Work out the finished part from the listing and answer in its coordinate system (mm). A direction names the side the tool comes from. Round coordinates to 2 decimals unless told otherwise and drop trailing zeros. Loops run counter-clockwise (first coordinate to the right, second up) from the corner with the lowest first, then second, coordinate; pieces in that order, holes last.
from build123d import *

# Parameters (mm, degrees)
F3_D = 6.3
F5_D = 6.3


with BuildPart() as f1:
    # F0 (on Front) → F1 (revolve)
    with BuildSketch(Plane.XZ):
        Polygon((-47.65, 6.3), (-47.65, 0), (-3.15, 0), (-3.15, 12.6), (-49.55, 12.6), (-49.55, 6.3), align=None)
    revolve(axis=Axis((0, 0, -5.1516543608), (0, 0, -1)))

    # F3 (through all)
    with Locations(Plane(origin=(0, 0, 0), x_dir=(1, 0, 0), z_dir=(0, 0, -1))):
        with Locations((25, 0), (-25, 0)):
            Hole(F3_D / 2)

    # F5 (through all)
    with Locations(Plane(origin=(0, 0, 0), x_dir=(1, 0, 0), z_dir=(0, 0, -1))):
        with Locations((-14, -20), (14, -20)):
            Hole(F5_D / 2)


solid = f1.part
Item 1: Straight lines are drawn through the part: line 1 (Y direction, x = 0, z = 4.5); line 2 (X direction, y = 0.5, z = 3); line 3 (X direction, y = 20, z = 4.5). For each, find the intervals that lie inside material, in ascending order.
Item 2: Determine the mould class of faces 1 (the face through (-45.45, 14.31, 3.11)), 2 (the face through (1, -10, 0)), 3 (the face through (2.5, -1.917, 6.388)), 4 (the face through (-21.853, -0.138, 6.388)) for opening direction X: pulls with the +X half, pulls with the -X half, needs draft (parallel to the pull), parting line crosses it, or undercut.
Item 3: Section C-C, the plane z = 4.5 is taken. Give the vertices of the cut face in (x, y).
Item 4: Section A-A, the plane x = 0 is taken. Give the vertices of the cut face in (y, z), plus the area to 3 significant figures.
Item 5: Section B-B, the plane y = 0 is taken. Give the vertices of the cut face in (x, z), plus the area to 3 significant figures.
Item 6: Each of these flat-tipped pins is pushed along its axis until it touches: P1, Ø2, axis at x = -31.5, z = 2, coming from the -Y side; P2, Ø1.5, axis at x = 19.5, z = 4.5, coming from the +Y side; P3, Ø4, axis at x = 14, z = 5.5, coming from the -Y side. Where does it stop, or does it pass through?
Item 7: Section D-D, the plane y = 20 is taken. Give the vertices of the cut face in (x, z), plus the area to 3 significant figures.
Item 8: For faces 5 (the face through (-11.5, 21.917, 6.388)), 6 (the face through (26, 41, 6.3)), determine the directions among +Z, -Z, +X, -X, +Y, -Y from which every point of the face is accessible in a straight line to the end or side of a thin tool.
Answer below:
1. line 1: y = -47.65 to -3.15, 3.15 to 47.65
1. line 2: x = -47.65 to -28.11, -21.89 to -3.11, 3.11 to 21.89, 28.11 to 47.65
1. line 3: x = -43.25 to -17.15, -10.85 to 10.85, 17.15 to 43.25
2. face 1: parting line crosses it
2. face 2: needs draft
2. face 3: undercut
2. face 4: undercut
3. outline: circle Ø95.3 at (0, 0); hole circle Ø6.3 at (-25, 0); hole circle Ø6.3 at (-14, 20); hole circle Ø6.3 at (0, 0); hole circle Ø6.3 at (14, 20); hole circle Ø6.3 at (25, 0)
4. outline: (-49.55, 6.3) - (-47.65, 6.3) - (-47.65, 0) - (-3.15, 0) - (-3.15, 12.6) - (-49.55, 12.6) - close; (3.15, 0) - (47.65, 0) - (47.65, 6.3) - (49.55, 6.3) - (49.55, 12.6) - (3.15, 12.6) - close
4. area: 1,150 mm2
5. outline: (-49.55, 6.3) - (-47.65, 6.3) - (-47.65, 0) - (-28.15, 0) - (-28.15, 12.6) - (-49.55, 12.6) - close; (-21.85, 0) - (-3.15, 0) - (-3.15, 12.6) - (-21.85, 12.6) - close; (3.15, 0) - (21.85, 0) - (21.85, 12.6) - (3.15, 12.6) - close; (28.15, 0) - (47.65, 0) - (47.65, 6.3) - (49.55, 6.3) - (49.55, 12.6) - (28.15, 12.6) - close
5. area: 987 mm2
6. P1: stops at y = -36.61
6. P2: stops at y = 43.81
6. P3: stops at y = -48.03
7. outline: (-45.33, 6.3) - (-43.25, 6.3) - (-43.25, 0) - (-17.15, 0) - (-17.15, 12.6) - (-45.33, 12.6) - close; (-10.85, 0) - (10.85, 0) - (10.85, 12.6) - (-10.85, 12.6) - close; (17.15, 0) - (43.25, 0) - (43.25, 6.3) - (45.33, 6.3) - (45.33, 12.6) - (17.15, 12.6) - close
7. area: 957 mm2
8. face 5: +Z, -Z
8. face 6: -Z
